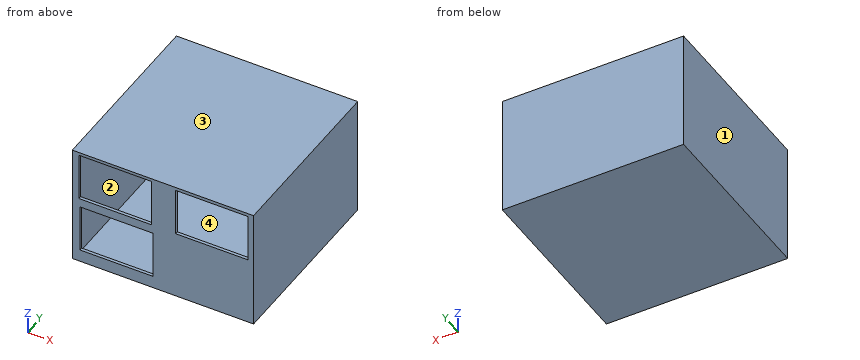
```python
from build123d import *

# Parameters (mm, degrees)
F0_W     = 150
F0_H     = 100
F1_DEPTH = 150
F2_T     = -2.5
F3_W     = 60
F3_H     = 40
F4_DEPTH = 468.9
F5_W     = 60
F5_H     = 40
F6_DEPTH = 145
F7_W     = 60.590963345
F7_H     = 39.7856272757
F8_DEPTH = 146.1


# Not quite as in the source:
# - a feature names something its author has since deleted; it is built from what else it names


with BuildPart() as f1:
    # F0 (on Right) → F1 (new body)
    with BuildSketch(Plane.YZ):
        with Locations((-13.7818545103, -23.5450232641)):
            Rectangle(F0_W, F0_H)
    extrude(amount=F1_DEPTH)

    # F2 (hollow: no face is removed)
    offset(amount=F2_T, mode=Mode.SUBTRACT)

    # F3 (on Front) → F4 (cut)
    with BuildSketch(Plane.XZ):
        with Locations((35.4225549102, 3.9785955846)):
            Rectangle(F3_W, F3_H)
    extrude(amount=F4_DEPTH, mode=Mode.SUBTRACT)

    # F5 (on face) → F6 (cut)
    with BuildSketch(Plane.XZ.offset(88.7818545103)):
        with Locations((115.576479584, 3.7956100403)):
            Rectangle(F5_W, F5_H)
    extrude(amount=-F6_DEPTH, mode=Mode.SUBTRACT)

    # F7 (on face) → F8 (cut)
    with BuildSketch(Plane.XZ.offset(88.7818545103)):
        with Locations((36.6743972991, -43.25533472)):
            Rectangle(F7_W, F7_H)
    extrude(amount=-F8_DEPTH, mode=Mode.SUBTRACT)


solid = f1.part
```
Build history of the part. All positions in model axes, mm. Face numbers are marked on the shaded views. Coordinates: 2 decimals unless noted, no trailing zeros. Order: outer loops, then holes, each group sorted by start corner. A loop starts at its lowest first (then second) coordinate and runs counter-clockwise, first axis right, second up.
Item 1: Drop flat-ended pins along their axis: pin 1 Ø12 at (y, z) = (45.5, -31.5) entering from -X; pin 2 Ø1 at (x, z) = (24, -35) entering from -Y. Give the stop position or say it passes through.
Filled in:
pin 1: stops at x = 0
pin 2: stops at y = 58.72
Item 2: Mould opens along Z. For the marked faces 1, 2, 3 and 4 say: released by +Z, released by -Z, zero draft, split by the parting line, or undercut.
Filled in:
face 1: zero draft
face 2: undercut
face 3: released by +Z
face 4: undercut
Item 3: Drill centre lines: L1, parallel to X at y = 4.5, z = 7; L2, parallel to Z at x = 106, y = 45; L3, parallel to Y at x = 92, z = -42.5. Where is each one in solid material? Low to high.
Filled in:
L1: x = 0 to 2.5, 147.5 to 150
L2: z = -73.55 to -71.05, 23.95 to 26.45
L3: y = -88.78 to -86.28, 58.72 to 61.22
Item 4: Saw through at A-A on z = -9. List the corners of the cut face in (x, y).
Filled in:
outline: (0, -88.78) - (5.42, -88.78) - (5.42, -86.28) - (2.5, -86.28) - (2.5, 58.72) - (147.5, 58.72) - (147.5, -86.28) - (145.58, -86.28) - (145.58, -88.78) - (150, -88.78) - (150, 61.22) - (0, 61.22) - close; (65.42, -88.78) - (85.58, -88.78) - (85.58, -86.28) - (65.42, -86.28) - close
Item 5: Saw through at B-B on x = 83. List the corners of the cut face in (y, z), then the cut area to 4 significant figures.
Filled in:
outline: (-88.78, -73.55) - (61.22, -73.55) - (61.22, 26.45) - (-88.78, 26.45) - close; hole (-86.28, -71.05) - (58.72, -71.05) - (58.72, 23.95) - (-86.28, 23.95) - close
area: 1,225 mm2
Item 6: Saw through at D-D on y = 18. List the corners of the cut face in (x, z), then the cut area to 4 significant figures.
Filled in:
outline: (0, -73.55) - (150, -73.55) - (150, 26.45) - (0, 26.45) - close; hole (2.5, -71.05) - (147.5, -71.05) - (147.5, 23.95) - (2.5, 23.95) - close
area: 1,225 mm2
